Verification items for the finished model (mm, model axes). A direction names the side the tool comes from. Round coordinates to 2 decimals unless told otherwise and drop trailing zeros. Loops run counter-clockwise (first coordinate to the right, second up) from the corner with the lowest first, then second, coordinate; pieces in that order, holes last. Notation, with made-up numbers: (85.5, 28.5) -> (117.5, 28.5) arc R17 cw to (117.5, 58.5) -> close; hole circle Ø9 at (42.5, 4.5). An arc over 180 degrees is marked (long way). Use a Markdown table: item, result. Add a question column.
```python
from build123d import *

# Parameters (mm, degrees)
F0_W     = 40
F0_H     = 14
F2_W     = 26.532998
F2_H     = 7.604173
F2_H_2   = 9.77986
F3_DEPTH = 5
F4_R     = 8
F5_DEPTH = 45
F6_R     = 3
F7_DEPTH = 5
F8_SIZE  = 0.5


with BuildPart() as f1:
    # F0 (on Right) → F1 (revolve)
    with BuildSketch(Plane.YZ):
        with Locations((20, 7)):
            Rectangle(F0_W, F0_H)
        Polygon((-5, 0), (0, 0), (0, 14), (0, 24), (-5, 24), align=None)
    revolve(axis=Axis((0, 20, 0), (0, 1, 0)))

    # F2 (on face) → F3 (cut)
    with BuildSketch(Plane.XZ.offset(5)):
        with Locations((0, 23.802087)):
            Rectangle(F2_W, F2_H)
        with Locations((0, -24.88993)):
            Rectangle(F2_W, F2_H_2)
    extrude(amount=-F3_DEPTH, mode=Mode.SUBTRACT)

    # F4 (on face) → F5 (cut)
    with BuildSketch(Plane.XZ.offset(5)):
        Circle(F4_R)
    extrude(amount=-F5_DEPTH, mode=Mode.SUBTRACT)

    # F6 (on face) → F7 (cut)
    with BuildSketch(Plane.XZ.offset(5)):
        with Locations((-13.435029, 13.435029)):
            Circle(F6_R)
        with Locations((13.435029, 13.435029)):
            Circle(F6_R)
        with Locations((13.435029, -13.435029)):
            Circle(F6_R)
        with Locations((-13.435029, -13.435029)):
            Circle(F6_R)
        with Locations((-19, 0)):
            Circle(F6_R)
        with Locations((19, 0)):
            Circle(F6_R)
    extrude(amount=-F7_DEPTH, mode=Mode.SUBTRACT)

    # F8
    f8_edges = [f1.edges().sort_by_distance(p)[0] for p in [
        (0, 40, -14),
    ]]
    chamfer(f8_edges, length=F8_SIZE)


solid = f1.part
```
1) Sectioned sample at C-C on z = -15.5. Enter the section's corners in (x, y), then the cut area to 3 significant figures.
2) Thickness scan on line 1 (Y direction, x = -5, z = -18); line 2 (Z direction, x = 17, y = -2); line 3 (X direction, y = -2, z = -4). Record the ranges inside material, lowest first.
3) Access from +Z, -Z, +X, -X, +Y, -Y to the whole of each face (thin tool, end or side, straight path). Record for faces 5 (the face through (-5.362, 20.026, 12.932)), 6 (the face through (-6, 40, -6)).
4) Release check for a two-part mould opening along Z. For faces 1 (the face through (11.22, -2.54, -11.41)), 2 (the face through (0, -3, 20)), 3 (the face through (-5, 0, 14)), 4 (the face through (-22, -3, 0)) record: released by +Z, released by -Z, zero draft, split by the parting line, or undercut.
5) Go/stop test with flat-tipped pins: pin 1 (18.5 mm diameter, centred on x = 0, z = 0, fed in from -Y); pin 2 (2 mm diameter, centred on y = 33.5, z = 1.5, fed in from -X); pin 3 (12 mm diameter, centred on x = -5, y = 15.5, fed in from -Z); pin 4 (8 mm diameter, centred on y = 8.5, z = 8.5, fed in from +X). Record where each tip stops, or that it passes through.
6) Sectioned sample at D-D on y = -1. Enter the section's corners in (x, z).
7) Sectioned sample at A-A on z = 0. Enter the section's corners in (x, y), then the cut area to 3 significant figures.
8) Sectioned sample at B-B on x = -19. Enter the section's corners in (y, z), then the cut area to 3 significant figures.
Geometry results:
| question | item | result |
|---|---|---|
| 1 | outline | (-18.32, -5) -> (-15.61, -5) -> (-15.61, 0) -> (-18.32, 0) -> close; (-11.26, -5) -> (11.26, -5) -> (11.26, 0) -> (-11.26, 0) -> close; (15.61, -5) -> (18.32, -5) -> (18.32, 0) -> (15.61, 0) -> close |
| 1 | area | 140 mm^2 |
| 2 | line 1 | -5 to 0 |
| 2 | line 2 | -16.94 to -2.24, 2.24 to 16.94 |
| 2 | line 3 | -23.66 to -6.93, 6.93 to 23.66 |
| 3 | face 5 | +Y |
| 3 | face 6 | +Z, -Z, +X, -X, +Y |
| 4 | face 1 | undercut |
| 4 | face 2 | released by +Z |
| 4 | face 3 | zero draft |
| 4 | face 4 | undercut |
| 5 | pin 1 | y = -5 |
| 5 | pin 2 | x = -13.99 |
| 5 | pin 3 | z = -14 |
| 5 | pin 4 | x = 13.26 |
| 6 | outline | (-13.27, -20) -> (13.27, -20) arc R24 ccw to (13.27, 20) -> (-13.27, 20) arc R24 ccw to start; hole circle Ø6 at (-19, 0); hole circle Ø6 at (-13.44, -13.44); hole circle Ø6 at (-13.44, 13.44); hole circle Ø16 at (0, 0); hole circle Ø6 at (13.44, -13.44); hole circle Ø6 at (13.44, 13.44); hole circle Ø6 at (19, 0) |
| 7 | outline | (-24, -5) -> (-22, -5) -> (-22, 0) -> (-24, 0) -> close; (-16, -5) -> (-8, -5) -> (-8, 40) -> (-13.5, 40) -> (-14, 39.5) -> (-14, 0) -> (-16, 0) -> close; (8, -5) -> (16, -5) -> (16, 0) -> (14, 0) -> (14, 39.5) -> (13.5, 40) -> (8, 40) -> close; (22, -5) -> (24, -5) -> (24, 0) -> (22, 0) -> close |
| 7 | area | 580 mm^2 |
| 8 | outline | (-5, -14.66) -> (0, -14.66) -> (0, -3) -> (-5, -3) -> close; (-5, 3) -> (0, 3) -> (0, 14.66) -> (-5, 14.66) -> close |
| 8 | area | 117 mm^2 |
